Autodesk Inventor part; units mm, degrees
ref_plane "YZ Plane" through (0, 0, 0) normal (1, 0, 0) x (0, 1, 0)
ref_plane "XZ Plane" through (0, 0, 0) normal (0, 1, 0) x (-1, 0, 0)
ref_plane "XY Plane" through (0, 0, 0) normal (0, 0, 1) x (1, 0, 0)
sketch "Sketch1" plane through (0, 0, 0) normal (0, 0, 1) x (1, 0, 0)
  line L0 (22.5, 33.5) -> (-22.5, 33.5)
  line L1 (-22.5, 33.5) -> (-22.5, -33.5)
  line L2 (-22.5, -33.5) -> (22.5, -33.5)
  line L3 (22.5, -33.5) -> (22.5, 33.5)
  line L4 (22.5, 33.5) -> (-22.5, -33.5) construction
  line L5 (-22.5, 33.5) -> (22.5, -33.5) construction
  line L6 (-18.25, 25.5) -> (18.25, 25.5) construction
  line L7 (18.25, 25.5) -> (18.25, -25.5) construction
  line L8 (18.25, -25.5) -> (-18.25, -25.5) construction
  line L9 (-18.25, -25.5) -> (-18.25, 25.5) construction
  line L10 (-18.25, 25.5) -> (18.25, -25.5) construction
  line L11 (18.25, 25.5) -> (-18.25, -25.5) construction
  line L12 (22.5, 0) -> (-22.5, 0) construction
  line L13 (0, 33.5) -> (0, -33.5) construction
  circle A0 centre (18.25, 25.5) radius 2.4
  circle A1 centre (-18.25, 25.5) radius 2.4
  circle A2 centre (18.25, -25.5) radius 2.4
  circle A3 centre (-18.25, -25.5) radius 2.4
  line L14 (18.25, 32.5) -> (18.25, 18.5) construction
  line L15 (21.5, 17.5) -> (-21.5, 17.5)
  line L16 (-21.5, 17.5) -> (-21.5, -17.5)
  line L17 (-21.5, -17.5) -> (21.5, -17.5)
  line L18 (21.5, -17.5) -> (21.5, 17.5)
  line L19 (21.5, 17.5) -> (-21.5, -17.5) construction
  line L20 (-21.5, 17.5) -> (21.5, -17.5) construction
  line L21 (14, 17.5) -> (14, 32.5)
  line L22 (14, 32.5) -> (-14, 32.5)
  line L23 (-14, 32.5) -> (-14, 17.5)
  line L24 (14, -17.5) -> (14, -32.5)
  line L25 (14, -32.5) -> (-14, -32.5)
  line L26 (-14, -32.5) -> (-14, -17.5)
  arc A4 (15.9605, 26.2199) -> (15.9605, 24.7801) centre (15.75, 25.5) ccw
  arc A5 (20.5395, 24.7801) -> (20.5395, 26.2199) centre (20.75, 25.5) ccw
  arc A6 (15.9605, -24.7801) -> (15.9605, -26.2199) centre (15.75, -25.5) ccw
  arc A7 (20.5395, -26.2199) -> (20.5395, -24.7801) centre (20.75, -25.5) ccw
  arc A8 (-15.9605, 24.7801) -> (-15.9605, 26.2199) centre (-15.75, 25.5) ccw
  arc A9 (-20.5395, 26.2199) -> (-20.5395, 24.7801) centre (-20.75, 25.5) ccw
  arc A10 (-15.9605, -26.2199) -> (-15.9605, -24.7801) centre (-15.75, -25.5) ccw
  arc A11 (-20.5395, -24.7801) -> (-20.5395, -26.2199) centre (-20.75, -25.5) ccw
  point P0 (0, 0)
  point P1 (14, -17.5)
  point P2 (-14, -17.5)
  point P3 (21.5, 25.5)
  point P4 (15, 25.5)
  point P5 (20.5395, 26.2199)
  point P6 (20.5395, 24.7801)
  point P7 (20.5395, -24.7801)
  point P8 (20.5395, -26.2199)
  point P9 (15.9605, -26.2199)
  point P10 (15.9605, -24.7801)
  point P11 (-20.5395, -26.2199)
  point P12 (-20.5395, -24.7801)
  point P13 (-15.9605, -24.7801)
  point P14 (-15.9605, -26.2199)
  point P15 (-20.5395, 24.7801)
  point P16 (-20.5395, 26.2199)
  point P17 (-15.9605, 26.2199)
  point P18 (-15.9605, 24.7801)
  dimension "d0" = 45
  dimension "d1" = 67
  dimension "d19" = 4.8
  dimension "d33" = 51
  dimension "d34" = 36.5
  dimension "d38" = 1
  dimension "d43" = 1
  dimension "d44" = 1
  dimension "d46" = 6.5
  dimension "d47" = 1.5
  dimension "d48" = 1
  dimension "d50" = 16
extrude "Extrusion1" add sketch "Sketch1" along normal blind 1.6 contours L3 L2 L1 L0 | L18 L17 L16 L15 | L15 L23 L22 L21 | L24 L25 L26 L17
extrude "Extrusion2" add sketch "Sketch1" along normal blind 31.6 contours L18 L17 L16 L15 | L15 L23 L22 L21 | L24 L25 L26 L17
fillet "Fillet1" radius 2 12 edges at (21.5, -17.5, 16.6) (21.5, 17.5, 16.6) (-21.5, -17.5, 16.6) (-21.5, 17.5, 16.6) (14, 17.5, 16.6) (14, -17.5, 16.6) (14, -32.5, 16.6) (-14, -32.5, 16.6) (-14, -17.5, 16.6) (-14, 17.5, 16.6) (-14, 32.5, 16.6) (14, 32.5, 16.6)
properties part number "SUSTAINA-RS485-COMMUNICATION-BOARD" material "Acetal Resin, Black"
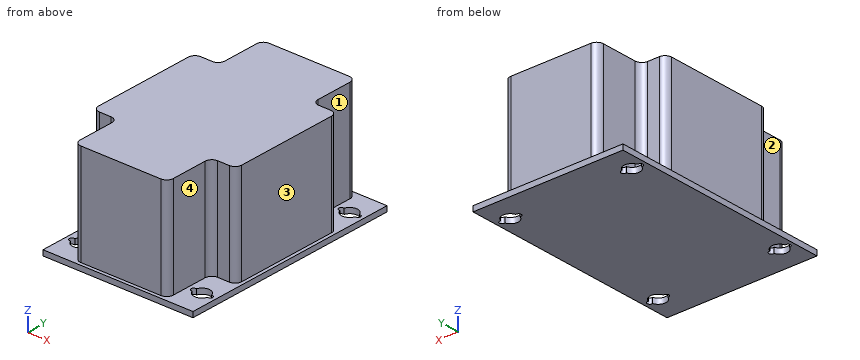
Geometry check sheet. Reference: the model listing, model coordinates, mm. Face numbers are marked on the shaded views. A direction names the side the tool comes from. Round coordinates to 2 decimals unless told otherwise and drop trailing zeros. Loops run counter-clockwise (first coordinate to the right, second up) from the corner with the lowest first, then second, coordinate; pieces in that order, holes last. Notation, with made-up numbers: (-24, -29) - (23, -29) arc R22 cw to (23, -2) - close; hole circle Ø7 at (-21, -2). An arc over 180 degrees is marked (long way). Write each question's results on one line, items separated by ' | '. Start each with the question number.
Q1. Cross-section at D-D on z = 17.5. Enter the section's corners in (x, y).
Q2. Cross-section at B-B on y = -9.5. Enter the section's corners in (x, z), and give its area (3 significant figures).
Q3. Gauge pin test, flat ends, axial feed: P1, Ø3.5, axis at y = -24.5, z = 19.5, coming from the -X side; P2, Ø6, axis at x = 10.5, y = -3.5, coming from the -Z side; P3, Ø3, axis at y = 6, z = 24.5, coming from the +X side; P4, Ø0.9, axis at x = 15.75, y = 25.5, coming from the +Z side. Record the tip position at first contact, or that the pin passes through.
Q4. Cross-section at C-C on x = -11. Enter the section's corners in (y, z).
Q5. Thickness scan on line 1 (Y direction, x = -15.75, z = 1.05); line 2 (X direction, y = 25, z = 1); line 3 (Y direction, x = -17, z = 7). Record the ranges inside material, lowest first. Write a range as [from, to].
Q6. Access from +Z, -Z, +X, -X, +Y, -Y to the whole of each face (thin tool, end or side, straight path). Record for the marked faces 1, 2, 3 and 4.
Q7. Cross-section at A-A on y = -25.5. Enter the section's corners in (x, z), and give its area (3 significant figures).
Answers below:
1) outline: (-21.5, -15.5) arc R2 ccw to (-19.5, -17.5) - (-16, -17.5) arc R2 cw to (-14, -19.5) - (-14, -30.5) arc R2 ccw to (-12, -32.5) - (12, -32.5) arc R2 ccw to (14, -30.5) - (14, -19.5) arc R2 cw to (16, -17.5) - (19.5, -17.5) arc R2 ccw to (21.5, -15.5) - (21.5, 15.5) arc R2 ccw to (19.5, 17.5) - (16, 17.5) arc R2 cw to (14, 19.5) - (14, 30.5) arc R2 ccw to (12, 32.5) - (-12, 32.5) arc R2 ccw to (-14, 30.5) - (-14, 19.5) arc R2 cw to (-16, 17.5) - (-19.5, 17.5) arc R2 ccw to (-21.5, 15.5) - close
2) outline: (-22.5, 0) - (22.5, 0) - (22.5, 1.6) - (21.5, 1.6) - (21.5, 31.6) - (-21.5, 31.6) - (-21.5, 1.6) - (-22.5, 1.6) - close | area: 1,360 mm²
3) P1: stops at x = -14 | P2: stops at z = 0 | P3: stops at x = 21.5 | P4: passes through
4) outline: (-33.5, 0) - (33.5, 0) - (33.5, 1.6) - (32.5, 1.6) - (32.5, 31.6) - (-32.5, 31.6) - (-32.5, 1.6) - (-33.5, 1.6) - close
5) line 1: y = [-33.5, -26.25], [-24.75, 24.75], [26.25, 33.5] | line 2: x = [-22.5, -21.31], [-15.19, 15.19], [21.31, 22.5] | line 3: y = [-17.5, 17.5]
6) face 1: +Z, +X, +Y | face 2: +Z, -X, -Y | face 3: +Z, +X, +Y, -Y | face 4: +Z, +X, -Y
7) outline: (-22.5, 0) - (-21.5, 0) - (-21.5, 1.6) - (-22.5, 1.6) - close; (-15, 0) - (15, 0) - (15, 1.6) - (14, 1.6) - (14, 31.6) - (-14, 31.6) - (-14, 1.6) - (-15, 1.6) - close; (21.5, 0) - (22.5, 0) - (22.5, 1.6) - (21.5, 1.6) - close | area: 891 mm²
